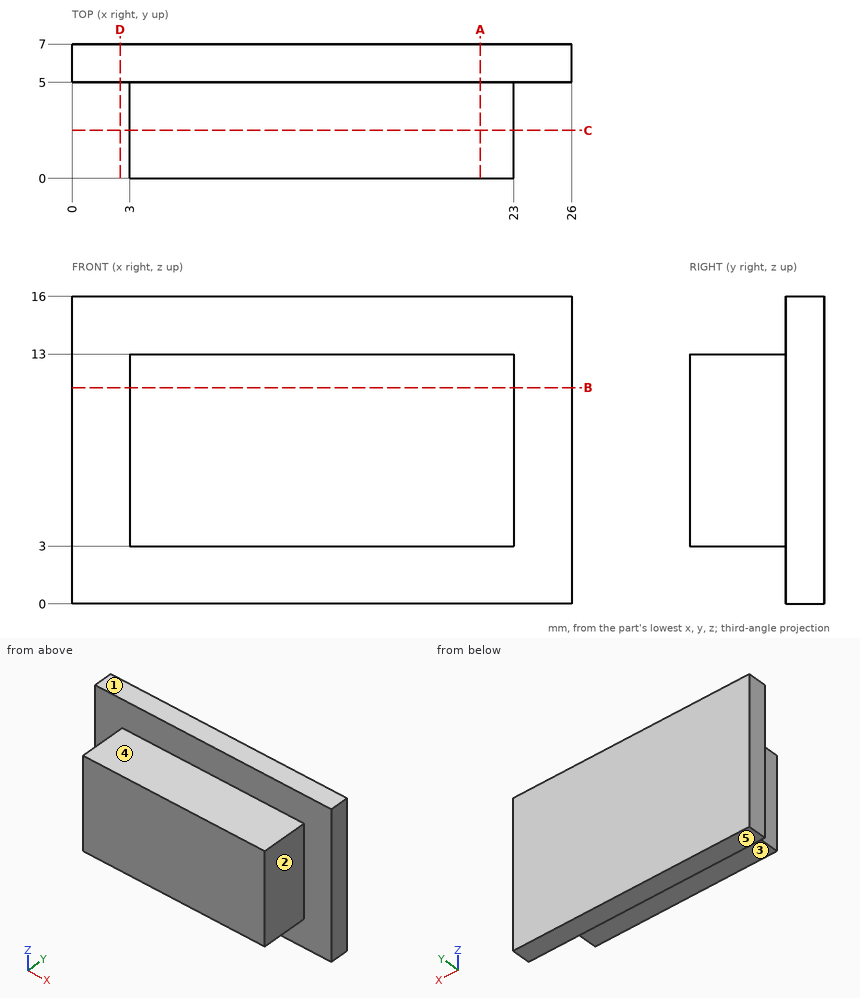
Drawing for the job (mm, zero at the part's lowest x, y, z). A direction names the side the tool comes from. Round coordinates to 2 decimals unless told otherwise and drop trailing zeros. Write each loop counter-clockwise with the first axis right and the second up, starting at its lowest first coordinate (ties: lowest second). Pieces come first, ordered by that corner, then holes. Notation, with made-up numbers: M 66,-22.5 L 80,-22.5 A18 cw 80,8.5 Z; hole C 1.5,5 d5. An arc over 180 degrees is marked long. Answer in a Markdown table with one row per item.
1. Probe L1, parallel to Z at x = 13.75, y = 3.75; L2, parallel to X at y = 3.25, z = 6.25; L3, parallel to Y at x = 15, z = 14. List the from-to ranges inside material, lowest first. Write a range as [from, to].
Geometry check:
| item | result |
|---|---|
| L1 | [3, 13] |
| L2 | [3, 23] |
| L3 | [5, 7] |
2. Saw through at A-A (x = 21.25). List the corners of the cut face in (y, z), and give its area (3 significant figures).
Geometry check:
| item | result |
|---|---|
| outline | M 0,3 L 5,3 L 5,0 L 7,0 L 7,16 L 5,16 L 5,13 L 0,13 Z |
| area | 82.0 mm2 |
3. Saw through at B-B (z = 11.25). List the corners of the cut face in (x, y), and give its area (3 significant figures).
Geometry check:
| item | result |
|---|---|
| outline | M 0,5 L 3,5 L 3,0 L 23,0 L 23,5 L 26,5 L 26,7 L 0,7 Z |
| area | 152 mm2 |
4. Saw through at C-C (y = 2.5). List the corners of the cut face in (x, z).
Geometry check:
| item | result |
|---|---|
| outline | M 3,3 L 23,3 L 23,13 L 3,13 Z |
5. Flat gauge pins, fed straight in: P1, Ø4, axis at y = 2.5, z = 10, coming from the +X side; P2, Ø2.5, axis at x = 10, y = 1.5, coming from the -Z side; P3, Ø4, axis at x = 8.5, y = 1, coming from the +Z side. Where does each tip first touch, or does it go through?
Geometry check:
| item | result |
|---|---|
| P1 | x = 23 |
| P2 | z = 3 |
| P3 | z = 13 |
6. Saw through at D-D (x = 2.5). List the corners of the cut face in (y, z).
Geometry check:
| item | result |
|---|---|
| outline | M 5,0 L 7,0 L 7,16 L 5,16 Z |
7. Which spindle directions (+Z, -Z, +X, -X, +Y, -Y) get a long thin tool onto all of the face, cutting with end or side? Do the marked faces 1, 2, 3, 4 and 5. Say none if no direction does.
Geometry check:
| item | result |
|---|---|
| face 1 | +Z, +X, -X, +Y, -Y |
| face 2 | +Z, -Z, +X, -Y |
| face 3 | -Z, +X, -X, -Y |
| face 4 | +Z, +X, -X, -Y |
| face 5 | -Z, +X, -X, +Y, -Y |
